Model file for the job. Use its own axes, mm. A direction names the side the tool comes from. Round coordinates to 2 decimals unless told otherwise and drop trailing zeros. Loops run counter-clockwise (first coordinate to the right, second up) from the corner with the lowest first, then second, coordinate; pieces in that order, holes last.
from build123d import *

# Parameters (mm, degrees)
SKETCH_1_R      = 1.65
SKETCH_1_W      = 272.523786307
SKETCH_1_H      = 131.563207183
EXTRUDE_4_DEPTH = 10


with BuildPart() as part:
    # 草图1 → 凸台-拉伸4 (new body)
    with BuildSketch(Plane.XY):
        with BuildLine():
            Line((-77.155190134, 109.874140248), (212.844809866, 109.874140248))
            ThreePointArc((212.844809866, 109.874140248), (216.380343772, 108.409674154), (217.844809866, 104.874140248))
            Line((217.844809866, 104.874140248), (217.844809866, -35.125859752))
            ThreePointArc((217.844809866, -35.125859752), (216.380343772, -38.661393658), (212.844809866, -40.125859752))
            Line((212.844809866, -40.125859752), (-77.155190134, -40.125859752))
            ThreePointArc((-77.155190134, -40.125859752), (-80.69072404, -38.661393658), (-82.155190134, -35.125859752))
            Line((-82.155190134, -35.125859752), (-82.155190134, 104.874140248))
            ThreePointArc((-82.155190134, 104.874140248), (-80.69072404, 108.409674154), (-77.155190134, 109.874140248))
        make_face()
        with Locations((-77.155190134, 104.874140248)):
            Circle(SKETCH_1_R, mode=Mode.SUBTRACT)
        with Locations((212.844809866, -35.125859752)):
            Circle(SKETCH_1_R, mode=Mode.SUBTRACT)
        with Locations((-77.155190134, -35.125859752)):
            Circle(SKETCH_1_R, mode=Mode.SUBTRACT)
        with Locations((212.844809866, 104.874140248)):
            Circle(SKETCH_1_R, mode=Mode.SUBTRACT)
        with Locations((67.844809867, 34.874140248)):
            Rectangle(SKETCH_1_W, SKETCH_1_H, mode=Mode.SUBTRACT)
    extrude(amount=EXTRUDE_4_DEPTH)


solid = part.part
Q1. Probe line 1 (Y direction, x = -65, z = 8); line 2 (X direction, y = 94.5, z = 6). List the from-to ranges inside material, lowest first.
Q2. Pull direction Y, two halves, no side cores. Call faces 1 (the face through (-68.417, 34, 5)), 2 (the face through (-82.155, 34, 5)), 3 (the face through (66, -30.907, 5)), 4 (the face through (70, -40.126, 5)): pulls with the +Y half, pulls with the -Y half, needs draft (parallel to the pull), parting line crosses it, or undercut.
Q3. Slice it at C-C on z = 3.5. Give the cut face in (x, y).
Q4. Slice it at A-A on y = 58.5. Give the cut face in (x, z).
Q5. Tool access for faces 5 (the face through (79.7, -31.4, 0)), 6 (the face through (66, 100.656, 5)): list every direction of +Z, -Z, +X, -X, +Y, -Y with a clear straight run to the whole face (end or side of a thin tool).
Q6. Slice it at B-B on x = 16. Give the cut face in (y, z).
Reply:
1. line 1: y = -40.13 to -30.91, 100.66 to 109.87
1. line 2: x = -82.16 to -68.42, 204.11 to 217.84
2. face 1: undercut
2. face 2: needs draft
2. face 3: undercut
2. face 4: pulls with the -Y half
3. outline: (-82.16, -35.13) arc R5 ccw to (-77.16, -40.13) - (212.84, -40.13) arc R5 ccw to (217.84, -35.13) - (217.84, 104.87) arc R5 ccw to (212.84, 109.87) - (-77.16, 109.87) arc R5 ccw to (-82.16, 104.87) - close; hole circle Ø3.3 at (-77.16, -35.13); hole circle Ø3.3 at (-77.16, 104.87); hole (-68.42, -30.91) - (204.11, -30.91) - (204.11, 100.66) - (-68.42, 100.66) - close; hole circle Ø3.3 at (212.84, -35.13); hole circle Ø3.3 at (212.84, 104.87)
4. outline: (-82.16, 0) - (-68.42, 0) - (-68.42, 10) - (-82.16, 10) - close; (204.11, 0) - (217.84, 0) - (217.84, 10) - (204.11, 10) - close
5. face 5: -Z, +X, -X, +Y, -Y
5. face 6: +Z, -Z
6. outline: (-40.13, 0) - (-30.91, 0) - (-30.91, 10) - (-40.13, 10) - close; (100.66, 0) - (109.87, 0) - (109.87, 10) - (100.66, 10) - close
